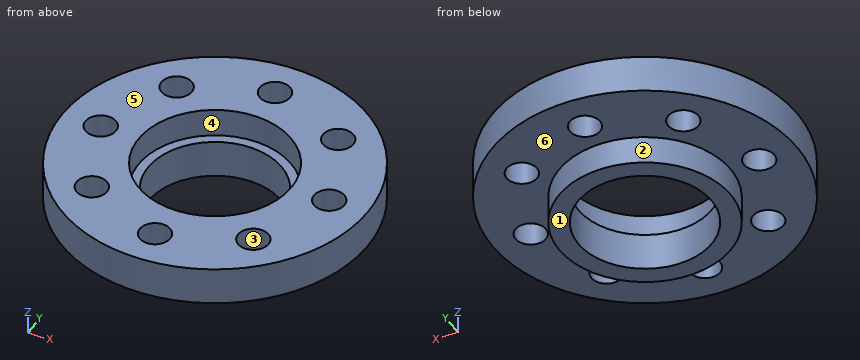
from build123d import *

# Parameters (mm, degrees)
F0_R     = 4.5
F0_R_2   = 3.5
F1_DEPTH = 1.5
F2_R     = 8
F2_R_2   = 0.8
F2_R_3   = 4.5
F2_R_4   = 3.5
F3_DEPTH = 2
F4_R     = 4
F5_DEPTH = 1.5


with BuildPart() as f1:
    # F0 (on Top) → F1 (new body)
    with BuildSketch(Plane.XY):
        Circle(F0_R)
        Circle(F0_R_2, mode=Mode.SUBTRACT)
    extrude(amount=F1_DEPTH)

    # F2 (on face) → F3 (join)
    with BuildSketch(Plane.XY.offset(1.5)):
        Circle(F2_R)
        with Locations((-4.2426406871, -4.2426406871)):
            Circle(F2_R_2, mode=Mode.SUBTRACT)
        with Locations((0, -6)):
            Circle(F2_R_2, mode=Mode.SUBTRACT)
        with Locations((4.2426406871, -4.2426406871)):
            Circle(F2_R_2, mode=Mode.SUBTRACT)
        with Locations((-6, 0)):
            Circle(F2_R_2, mode=Mode.SUBTRACT)
        with Locations((-4.2426406871, 4.2426406871)):
            Circle(F2_R_2, mode=Mode.SUBTRACT)
        Circle(F2_R_3, mode=Mode.SUBTRACT)
        with Locations((6, 0)):
            Circle(F2_R_2, mode=Mode.SUBTRACT)
        with Locations((0, 6)):
            Circle(F2_R_2, mode=Mode.SUBTRACT)
        with Locations((4.2426406871, 4.2426406871)):
            Circle(F2_R_2, mode=Mode.SUBTRACT)
        Circle(F2_R_3)
        Circle(F2_R_4, mode=Mode.SUBTRACT)
    extrude(amount=F3_DEPTH)

    # F4 (on face) → F5 (cut)
    with BuildSketch(Plane.XY.offset(3.5)):
        Circle(F4_R)
    extrude(amount=-F5_DEPTH, mode=Mode.SUBTRACT)


solid = f1.part
The listing builds one solid part. Answer for the finished solid, in the listing's coordinates (mm). Face numbers are marked on the shaded views. A direction names the side the tool comes from. Coordinates: 2 decimals unless noted, no trailing zeros. Write each loop counter-clockwise with the first axis right and the second up, starting at its lowest first coordinate (ties: lowest second). Pieces come first, ordered by that corner, then holes. Notation, with made-up numbers: M 14,34.5 L 25,34.5 A18 cw 25,67.5 Z; hole C 24.25,13 d4. An arc over 180 degrees is marked long. Put each result on its own line as item: value. Start each with the question number.
1. Flat-ended cylindrical pins translate along their axes: P1, Ø1.5, axis at x = -4.5, z = 1.5, coming from the +Y side; P2, Ø2.5, axis at x = -4.24, y = 4.24, coming from the -Z side; P3, Ø1, axis at y = 5.5, z = 2.5, coming from the -X side (3 decimals). Find the tip coordinate at first contact, or state that the pin passes through.
2. For a pull along X with two mould halves and no side action, classify the marked faces 1, 2 and 3 as pulls with the +X half, pulls with the -X half, needs draft (parallel to the pull), parting line crosses it, or undercut.
3. Which of the six approach directions +Z, -Z, +X, -X, +Y, -Y give full straight-line access (tool end or side, diameter ignored) to the marked faces 4, 5 and 6?
4. A cutting plane is placed at C-C on x = 4.75. Write down the section's boundary in (y, z).
5. Consider line 1 (Y direction, x = 0, z = 2.25); line 2 (Y direction, x = 3.75, z = 1.6); line 3 (Z direction, x = 7.25, y = 2.5). Determine where each line is inside the solid, lowest interval first. Write a range as from..to.
6. A cutting plane is placed at A-A on x = 1.5. Write down the section's boundary in (y, z).
Resolved:
1. P1: stops at y = 7.07
1. P2: stops at z = 1.5
1. P3: stops at x = -6.245
2. face 1: needs draft
2. face 2: parting line crosses it
2. face 3: undercut
3. face 4: +Z
3. face 5: +Z, +X, -X, +Y, -Y
3. face 6: -Z
4. outline: M -6.44,1.5 L -4.86,1.5 L -4.86,3.5 L -6.44,3.5 Z; M -3.62,1.5 L 3.62,1.5 L 3.62,3.5 L -3.62,3.5 Z; M 4.86,1.5 L 6.44,1.5 L 6.44,3.5 L 4.86,3.5 Z
5. line 1: y = -8..-6.8, -5.2..-4, 4..5.2, 6.8..8
5. line 2: y = -7.07..-4.87, -3.61..3.61, 4.87..7.07
5. line 3: z = 1.5..3.5
6. outline: M -7.86,1.5 L -4.24,1.5 L -4.24,0 L -3.16,0 L -3.16,2 L -3.71,2 L -3.71,3.5 L -7.86,3.5 Z; M 3.16,0 L 4.24,0 L 4.24,1.5 L 7.86,1.5 L 7.86,3.5 L 3.71,3.5 L 3.71,2 L 3.16,2 Z
